Verification items for the finished model (mm, model axes). A direction names the side the tool comes from. Round coordinates to 2 decimals unless told otherwise and drop trailing zeros. Write each loop counter-clockwise with the first axis right and the second up, starting at its lowest first coordinate (ties: lowest second). Pieces come first, ordered by that corner, then holes. Notation, with made-up numbers: M 19.25,85.25 L 49.25,85.25 A11 ccw 49.25,102.25 Z; hole C -0.75,3 d4. An arc over 180 degrees is marked long. One line per item, written item: value. Start each with the question number.
Item 1: Section check D-D, the plane z = -29.5. Record the cut outline in (x, y), then the cut area to 3 significant figures.
Item 2: Gauge pin test, flat ends, axial feed: pin 1 (5 mm diameter, centred on x = 19, z = -5, fed in from +Y); pin 2 (2.5 mm diameter, centred on x = 19, z = -5, fed in from +Y); pin 3 (3.5 mm diameter, centred on x = 71, z = -10, fed in from +Y). Record the tip position at first contact, or that the pin passes through.
Item 3: Section check A-A, the plane y = 7.5. Record the cut outline in (x, z), then the cut area to 3 significant figures.
Item 4: Thickness scan on probe 1 along Z at (x, y) = (71, 7.55); probe 2 along Z at (x, y) = (71, 4.5); probe 3 along Z at (x, y) = (19, 4.9). Record the ranges inside material, lowest first. Write a range as from..to.
Item 5: Tool access check on faces 5 (the face through (0, 2, -30)), 6 (the face through (69, 5.8, -38)). Record the directions out of +Z, -Z, +X, -X, +Y, -Y that give a thin tool (end or side, any length) a straight path to the whole face; none if there is none.
Item 6: Section check B-B, the plane z = -38.2. Record the cut outline in (x, y).
Item 7: Draft check along Z on faces 1 (the face through (40, 2, -58.4)), 2 (the face through (21.146, 7.929, -5.676)), 3 (the face through (71, 3.8, -38)), 4 (the face through (73, 10, -8)). Enter one of: +Z half, -Z half, draft (parallel to the pull), parting line (faces both ways), or undercut.
Autodesk Inventor part; units mm, degrees
ref_plane "YZ Plane" through (0, 0, 0) normal (1, 0, 0) x (0, 1, 0)
ref_plane "XZ Plane" through (0, 0, 0) normal (0, 1, 0) x (-1, 0, 0)
ref_plane "XY Plane" through (0, 0, 0) normal (0, 0, 1) x (1, 0, 0)
sketch "Sketch1" plane through (0, 0, 0) normal (0, 1, 0) x (-1, 0, 0)
  line L0 (0, 0) -> (-78.6, 0)
  line L1 (-78.6, 0) -> (-78.6, -58.4)
  line L2 (-78.6, -58.4) -> (0, -58.4)
  line L3 (0, -58.4) -> (0, 0)
  dimension "d0" = 78.6
  dimension "d1" = 58.4
extrude "Extrusion1" add sketch "Sketch1" along normal blind 5
sketch "Sketch2" plane through (0, 5, 0) normal (0, 1, 0) x (1, 0, 0)
  circle A0 centre (19, 5) radius 4
  line L0 (0, 58.4) -> (0, 0)
  line L1 (0, 0) -> (78.6, 0)
  circle A1 centre (20.2, 53.4) radius 4
  line L2 (78.6, 58.4) -> (0, 58.4)
  circle A2 centre (71, 38.2) radius 4
  circle A3 centre (71, 10.2) radius 4
  line L3 (78.6, 0) -> (78.6, 58.4)
  dimension "d4" = 8
  dimension "d5" = 19
  dimension "d6" = 5
  dimension "d7" = 8
  dimension "d8" = 20.2
  dimension "d9" = 5
  dimension "d10" = 8
  dimension "d11" = 8
  dimension "d12" = 20.2
  dimension "d13" = 7.6
  dimension "d14" = 7.6
  dimension "d15" = 28
extrude "Extrusion2" add sketch "Sketch2" along normal blind 5 contours A0 | A1 | A2 | A3
sketch "Sketch3" plane through (20.2, 10, -53.4) normal (0, 1, 0) x (1, 0, 0)
  circle A0 centre (50.8, -15.2) radius 4
  circle A1 centre (0, 0) radius 4
  circle A2 centre (-1.2, -48.4) radius 4
  circle A3 centre (50.8, -43.2) radius 4
  circle A4 centre (0, 0) radius 2.25
  circle A5 centre (50.8, -15.2) radius 2.25
  circle A6 centre (-1.2, -48.4) radius 2.25
  circle A7 centre (50.8, -43.2) radius 2.25
  point P0 (-20.2, -53.4)
  dimension "d18" = 4.5
  dimension "d19" = 4.5
  dimension "d20" = 4.5
  dimension "d21" = 4.5
extrude "Extrusion3" cut sketch "Sketch3" against normal blind 4.2 contours A4 | A5 | A6 | A7
sketch "Sketch4" plane through (20.2, 5.8, -53.4) normal (0, 1, 0) x (1, 0, 0)
  circle A0 centre (0, 0) radius 2.25
  circle A1 centre (50.8, -15.2) radius 2.25
  circle A2 centre (50.8, -43.2) radius 2.25
  circle A3 centre (-1.2, -48.4) radius 2.25
  circle A4 centre (0, 0) radius 1.6
  circle A5 centre (50.8, -15.2) radius 1.6
  circle A6 centre (50.8, -43.2) radius 1.6
  circle A7 centre (-1.2, -48.4) radius 1.6
  point P0 (-20.2, -53.4)
  dimension "d24" = 3.2
  dimension "d25" = 3.2
  dimension "d26" = 3.2
  dimension "d27" = 3.2
extrude "Extrusion4" cut sketch "Sketch4" against normal blind 2 contours A4 | A5 | A6 | A7
chamfer "Chamfer1" distance 0.5 angle 45 4 edges at (16.2, 5, -53.4) (15, 5, -5) (67, 5, -10.2) (67, 5, -38.2)
fillet "Fillet1" radius 2 4 edges at (0, 2.5, -58.4) (0, 2.5, 0) (78.6, 2.5, 0) (78.6, 2.5, -58.4)
properties part number "Leonardo_Backplate"
Response values:
1. outline: M 0,0 L 78.6,0 L 78.6,5 L 0,5 Z
1. area: 393 mm2
2. pin 1: stops at y = 10
2. pin 2: stops at y = 3.8
2. pin 3: stops at y = 5.8
3. outline: C 19,-5 d8; C 20.2,-53.4 d8; C 71,-38.2 d8; C 71,-10.2 d8; hole C 19,-5 d4.5; hole C 20.2,-53.4 d4.5; hole C 71,-38.2 d4.5; hole C 71,-10.2 d4.5
3. area: 137 mm2
4. probe 1: z = -42.2..-40.45, -35.95..-34.2, -14.2..-12.45, -7.95..-6.2
4. probe 2: z = -58.4..-39.8, -36.6..-11.8, -8.6..0
4. probe 3: z = -58.4..-54.46, -52.34..-6.6, -3.4..0
5. face 5: +Z, -Z, -X, +Y, -Y
5. face 6: +Y
6. outline: M 0,0 L 78.6,0 L 78.6,5 L 75.5,5 L 75,5.5 L 75,10 L 73.25,10 L 73.25,5.8 L 72.6,5.8 L 72.6,3.8 L 69.4,3.8 L 69.4,5.8 L 68.75,5.8 L 68.75,10 L 67,10 L 67,5.5 L 66.5,5 L 0,5 Z
7. face 1: -Z half
7. face 2: undercut
7. face 3: undercut
7. face 4: draft
